Source: CAD feature listing. Evaluate the final solid. Frame: model axes, mm. Face numbers are marked on the shaded views. A direction names the side the tool comes from. Give positions to 0.01 mm unless a question says otherwise; leave off trailing zeros. Loops run counter-clockwise (first coordinate to the right, second up) from the corner with the lowest first, then second, coordinate; pieces in that order, holes last. Notation, with made-up numbers: (1, 37.25) - (17, 37.25) arc R18 cw to (17, 68.25) - close; hole circle Ø11 at (63.5, -6). An arc over 180 degrees is marked (long way). Write each question's results on one line, items separated by ' | '. Start each with the question number.
(1) Material intervals for line 1 along Y through (x, z) = (13.75, 0.7); line 2 along Z through (x, y) = (2.75, 0.15), sorted ascending. Write a range as [from, to].
(2) Cut plane A-A on x = 9. Return the cut outline in (y, z), then the cut area to 3 significant figures.
(3) Contact query for flat-ended pins moving along their axis: pin 1 (1.5 mm diameter, centred on x = 11, y = 1, fed in from -Z); pin 2 (3 mm diameter, centred on x = 9, z = 1.5, fed in from -Y); pin 3 (3 mm diameter, centred on x = 3, y = -2, fed in from -Z). Output: stop coordinate, or through.
(4) Pull-direction query (Y, two-part tool) for the marked faces 4, 5 and 6; classes: pulls with the +Y half, pulls with the -Y half, needs draft (parallel to the pull), parting line crosses it, or undercut.
(5) Reachability of the marked faces 1, 2 and 3 from +Z, -Z, +X, -X, +Y, -Y: full face, straight path, thin tool, end or side. Return the list, or none.
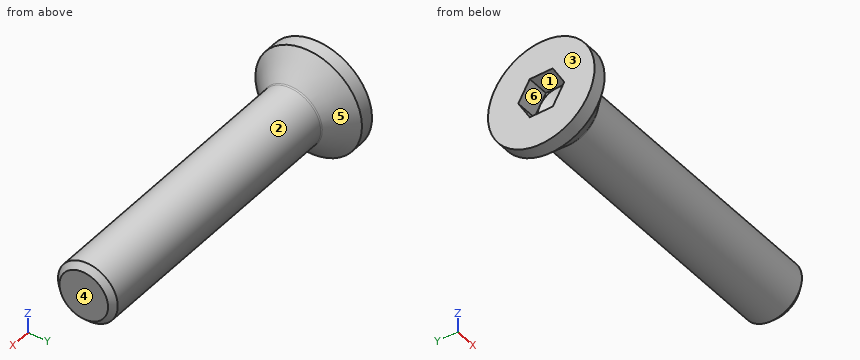
from build123d import *

# Parameters (mm, degrees)
FILLET1_R   = 0.1
HEX_START   = -1.1
HEX_2_DEPTH = 1.1


with BuildPart() as part:
    # BodySke → BaseBody (revolve)
    with BuildSketch(Plane.XY, mode=Mode.PRIVATE) as basebody_sk:
        Polygon((0, 0), (0, 2.675), (0.685, 2.675), (1.86, 1.5), (15.7195, 1.5), (16, 1.2195), (16, 0), align=None)
    revolve(basebody_sk.sketch.rotate(Axis((0, 0, 0), (1, 0, 0)), 90), axis=Axis((0, 0, 0), (1, 0, 0)))

    # Fillet1
    fillet1_edges = [part.edges().sort_by_distance(p)[0] for p in [
        (1.86, 0, -1.5),
    ]]
    fillet(fillet1_edges, radius=FILLET1_R)

    # Hex 2: read off the stored shape, not the designer's step
    # Hex 2 outline → Hex 2 (cut)
    with BuildSketch(Plane.ZY.offset(HEX_START)):
        Polygon((-1, -0.577350269), (0, -1.154700538), (1, -0.577350269), (1, 0.577350269), (0, 1.154700538), (-1, 0.577350269), align=None)
    extrude(amount=HEX_2_DEPTH, mode=Mode.SUBTRACT)

    # Hex 2 2 outline → Hex 2 2 (revolve, cut)
    with BuildSketch(Plane.YX):
        Polygon((1, 1.1), (0, 1.677350269), (0, 1.1), align=None)
    revolve(axis=Axis((0, 0, 0), (1, 0, 0)), mode=Mode.SUBTRACT)


solid = part.part
Ans:
1) line 1: [-1.33, 1.33] | line 2: [-1.49, 1.49]
2) outline: circle Ø3 at (0, 0) | area: 7.07 mm^2
3) pin 1: z = -1.48 | pin 2: y = -1.5 | pin 3: z = -1.41
4) face 4: needs draft | face 5: parting line crosses it | face 6: undercut
5) face 1: -X | face 2: +X | face 3: +Z, -Z, -X, +Y, -Y
